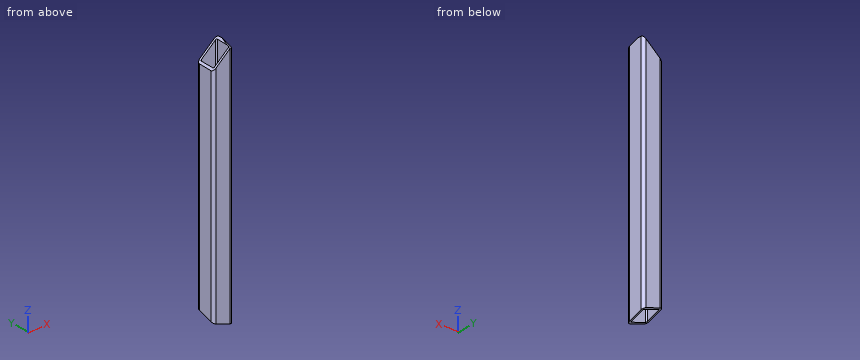
Autodesk Inventor part; units mm, degrees
ref_plane "Start Plane" through (0, 0, 4.614) normal (0, 0, 1) x (1, 0, 0)
ref_plane "End Plane" through (0, 0, 255.3168) normal (0, 0, 1) x (1, 0, 0)
ref_plane "Work Plane4" through (10.1657, 0, 255.4635) normal (-0.6628, 0, 0.7488) x (0.7488, 0, 0.6628)
ref_plane "Start Plane" through (0, 0, 4.614) normal (0, 0, 1) x (1, 0, 0)
ref_plane "End Plane" through (0, 0, 255.3168) normal (0, 0, 1) x (1, 0, 0)
sketch "Sketch" plane through (0, 0, 0) normal (0, 0, 1) x (1, 0, 0)
  line L0 (-10, -7) -> (-10, 7)
  line L1 (-7, 10) -> (7, 10)
  line L2 (10, 7) -> (10, -7)
  line L3 (7, -10) -> (-7, -10)
  arc A0 (-10, -7) -> (-7, -10) centre (-7, -7) ccw
  arc A1 (-7, 10) -> (-10, 7) centre (-7, 7) ccw
  arc A2 (10, 7) -> (7, 10) centre (7, 7) ccw
  arc A3 (7, -10) -> (10, -7) centre (7, -7) ccw
  arc A4 (-7, 8) -> (-8, 7) centre (-7, 7) ccw
  line L4 (-7, 8) -> (7, 8)
  arc A5 (8, 7) -> (7, 8) centre (7, 7) ccw
  line L5 (8, 7) -> (8, -7)
  arc A6 (7, -8) -> (8, -7) centre (7, -7) ccw
  line L6 (7, -8) -> (-7, -8)
  arc A7 (-8, -7) -> (-7, -8) centre (-7, -7) ccw
  line L7 (-8, -7) -> (-8, 7)
  line L8 (0, 14.8698) -> (0, -14.8698) construction
  line L9 (-14.8698, 0) -> (14.8698, 0) construction
  dimension "d7" = 3
  dimension "d10" = 20
  dimension "d11" = 20
  dimension "d12" = 2
  dimension "d15" = 10
  dimension "d16" = 10
extrude "Body" add sketch "Sketch" along normal up to surface (250.7028 mm away) from surface at 4.614
sketch "Sketch3" plane through (0, 0, 0) normal (0, 0, 1) x (1, 0, 0)
  line L0 (0, 0) -> (10, 0)
ref_plane "Work Plane3" through (0, 0, 0) normal (0, -1, 0) x (1, 0, 0)
sketch "Sketch4" plane through (0, 0, 0) normal (0, -1, 0) x (1, 0, 0)
  line L0 (-2, 4.614) -> (12, 4.614)
  line L1 (-2, 255.3168) -> (12, 255.3168)
  dimension "d18" = 250.7028
ref_plane "Work Plane4" through (10.1657, 0, 255.4635) normal (-0.6628, 0, 0.7488) x (0.7488, 0, 0.6628)
split "Split1" plane through (10.1657, 0, 255.4635) removes the side toward (-0.6628, 0, 0.7488)
ref_plane "Work Plane8" through (3.7296, 4.0763, 257.6842) normal (0.3124, -0.267, 0.9117) x (0.949, 0.0436, -0.3124)
split "Split2" plane through (3.7296, 4.0763, 257.6842) removes the side toward (0.3124, -0.267, 0.9117)
ref_plane "Work Plane9" through (-284.1797, -10.0613, 105.397) normal (-0.3124, 0.267, -0.9117) x (-0.1048, 0.9442, 0.3124)
split "Split3" plane through (-284.1797, -10.0613, 105.397) removes the side toward (-0.3124, 0.267, -0.9117)
equation "\"d7\" = G_IR"
equation "\"d10\" = G_H"
equation "\"d11\" = G_W"
equation "\"d12\" = G_T"
equation "\"d15\" = 0.5 * d10"
equation "\"d16\" = 0.5 * d11"
equation "\"d3\" = G_L"
equation "\"G_W\" = 20"
equation "\"G_H\" = 20"
equation "\"G_T\" = 2"
equation "\"G_IR\" = 3"
equation "\"G_L\" = 250.12582"
equation "\"G_OFFSET_START\" = -4.61403"
equation "\"G_OFFSET_END\" = 8.51725"
equation "\"d13\" = -G_OFFSET_START"
equation "\"d14\" = G_OFFSET_END + B_L"
equation "\"B_L\" = 246.79957"
properties part number "ISO 12633-2 - 20x20x2 - 250,13" material "Steel, Mild"
Source: CAD feature listing. Evaluate the final solid. Frame: model axes, mm. Give positions to 0.01 mm unless a question says otherwise; leave off trailing zeros. Write each loop counter-clockwise with the first axis right and the second up, starting at its lowest first coordinate (ties: lowest second). Pieces come first, ordered by that corner, then holes. Notation, with made-up numbers: M -34,66.5 L 2,66.5 A21 ccw 2,98.5 Z; hole C -33,31.25 d3. An arc over 180 degrees is marked long. Return JSON: item names as keys, results as strings. Group by question number.
1) Ray query, L1, parallel to Y at x = -6, z = 180; L2, parallel to Y at x = 9, z = 219. Return the intervals inside material, ascending.
2) First-contact query: pin 1 Ø4 at (x, y) = (-7, 0) entering from -Z; pin 2 Ø3 at (y, z) = (8, 207) entering from +X; pin 3 Ø10 at (x, y) = (4.5, 2) entering from -Z; pin 4 Ø10 at (x, y) = (-6, -5) entering from +Z. Flat tips, straight axial feed; report the tip coordinate or a pass-through.
3) Cut plane C-C, the plane x = 2. Output: boundary loops of the cut face in (y, z).
4) Cut plane A-A, the plane z = 118.5. Output: boundary loops of the cut face in (x, y), then the cut area to 3 significant figures.
5) Cut plane B-B, the plane y = 0.5. Output: boundary loops of the cut face in (x, z).
Data:
{
 "1": {"L1": "y = -10 to -8, 8 to 10", "L2": "y = -9.24 to 9.24"},
 "2": {"pin 1": "stops at z = 13.2", "pin 2": "stops at x = 10", "pin 3": "stops at z = 7.76", "pin 4": "stops at z = 244.7"},
 "3": {"outline": "M -10,7.35 L -8,7.94 L -8,248.24 L -10,248.24 Z; M 8,12.63 L 10,13.21 L 10,248.24 L 8,248.24 Z"},
 "4": {"outline": "M -10,-7 A3 ccw -7,-10 L 7,-10 A3 ccw 10,-7 L 10,7 A3 ccw 7,10 L -7,10 A3 ccw -10,7 Z; hole M -8,-7 A1 ccw -7,-8 L 7,-8 A1 ccw 8,-7 L 8,7 A1 ccw 7,8 L -7,8 A1 ccw -8,7 Z", "area": "137 mm²"},
 "5": {"outline": "M -10,14.54 L -8,13.86 L -8,239.38 L -10,237.61 Z; M 8,8.37 L 10,7.69 L 10,254.49 L 9.33,254.72 L 8,253.55 Z"}
}
